The model under review builds one solid part; all positions refer to its coordinate system, in mm. A direction names the side the tool comes from. Coordinates: 2 decimals unless noted, no trailing zeros. Loops run counter-clockwise (first coordinate to the right, second up) from the corner with the lowest first, then second, coordinate; pieces in that order, holes last. Notation, with made-up numbers: (44, 3) - (49, 3) arc R22 cw to (49, 37) - close; hole circle Ø9 at (69, 69.5). An arc over 180 degrees is marked (long way). Use a Markdown table: item, result. Add a question column.
1) Clearance check with flat-ended pins moving along their axes: pin 1 (3 mm diameter, centred on x = -32.86, z = -52.86, fed in from -Y); pin 2 (2.5 mm diameter, centred on x = -2.8, z = -22.8, fed in from -Y); pin 3 (3 mm diameter, centred on x = -19.5, y = -46.5, fed in from +Z); pin 4 (24.5 mm diameter, centred on x = -0.5, z = -19.5, fed in from -Y). State where each tip first meets the part, or that it passes through.
2) Add section A-A, the plane x = 4.5. Give the boundary of the cut face in (y, z).
3) To check wall thickness, follow L1, parallel to X at y = -45.85, z = -27; L2, parallel to X at y = -44.6, z = -43.5; L3, parallel to Y at x = 3.5, z = -25.5. State the ranges of each line that lie inside material, in increasing order. Write a range as [from, to].
4) Add section B-B, the plane z = -20. Give the boundary of the cut face in (x, y).
5) Add section D-D, the plane z = -27. Give the boundary of the cut face in (x, y), and give its area (3 significant figures).
6) For faces 1 (the cylindrical face through (-5.189, -45.521, -25.505)), 2 (the cylindrical face through (8.1, -42.48, -21.85)), list the 3-axis set-ups (+Z, -Z, +X, -X, +Y, -Y) from which the entire face can be reached by the end or side of a thin tool; tool diameter is ignored.
7) Add section C-C, the plane y = -42.5. Give the number of separate pieces and of enclosed holes in the cut face, and give its area (3 significant figures).
8) The part is to be moulded in two halves that separate along X. For faces 3 (the flat face through (-7.152, -44.042, -42.708)), 4 (the cylindrical face through (8.479, -42.479, -12.934)), 5 (the cylindrical face through (10.105, -42.521, -9.553)), say which applies: pulls with the +X half, pulls with the -X half, needs draft (parallel to the pull), parting line crosses it, or undercut.
```python
from build123d import *

# Parameters (mm, degrees)
CYLINDER020_R             = 11.1
CYLINDER020_DEPTH         = 26
CYLINDER019_R             = 4
CYLINDER019_DEPTH         = 43
CYLINDER021_R             = 1
CYLINDER021_DEPTH         = 31
CYLINDER024_R             = 1
CYLINDER024_DEPTH         = 31
CYLINDER023_R             = 1
CYLINDER023_DEPTH         = 31
CYLINDER022_R             = 1
CYLINDER022_DEPTH         = 31
FUSION002_ROLL_ANGLE      = -90
FUSION003_PLACEMENT_ANGLE = 180
SKETCH_R                  = 5
SKETCH_R_2                = 1.75
PAD_DEPTH                 = 6
CUT_PITCH_ANGLE           = 90
CLONE017_PITCH_ANGLE      = -45


with BuildPart() as cylinder141:
    # Cylinder020 → Cylinder020 (new body)
    with BuildSketch(Plane(origin=(-3, 71, 73), x_dir=(0, 0, 1), z_dir=(0, -1, 0))):
        Circle(CYLINDER020_R)
    extrude(amount=CYLINDER020_DEPTH)


with BuildPart() as fusion001:
    # Cylinder019 → Cylinder019 (new body)
    with BuildSketch(Plane(origin=(-3, 66, 73), x_dir=(0, 0, 1), z_dir=(0, -1, 0))):
        Circle(CYLINDER019_R)
    extrude(amount=CYLINDER019_DEPTH)

    # Fusion001: union Cylinder141
    add(cylinder141.part)


with BuildPart() as cylinder096:
    # Cylinder021 → Cylinder021 (new body)
    with BuildSketch(Plane(origin=(-7.5, -11, 132), x_dir=(1, 0, 0), z_dir=(0, 0, 1))):
        Circle(CYLINDER021_R)
    extrude(amount=CYLINDER021_DEPTH)


with BuildPart() as cylinder146:
    # Cylinder024 → Cylinder024 (new body)
    with BuildSketch(Plane(origin=(0, -3.5, 132), x_dir=(1, 0, 0), z_dir=(0, 0, 1))):
        Circle(CYLINDER024_R)
    extrude(amount=CYLINDER024_DEPTH)


with BuildPart() as cylinder145:
    # Cylinder023 → Cylinder023 (new body)
    with BuildSketch(Plane(origin=(7.5, -11, 132), x_dir=(1, 0, 0), z_dir=(0, 0, 1))):
        Circle(CYLINDER023_R)
    extrude(amount=CYLINDER023_DEPTH)


with BuildPart() as fusion003:
    # Cylinder022 → Cylinder022 (new body)
    with BuildSketch(Plane(origin=(0, -18.5, 132), x_dir=(1, 0, 0), z_dir=(0, 0, 1))):
        Circle(CYLINDER022_R)
    extrude(amount=CYLINDER022_DEPTH)

    # Fusion002: union Cylinder096, Cylinder146, Cylinder145
    add(cylinder096.part)
    add(cylinder146.part)
    add(cylinder145.part)


with BuildPart() as fusion003_1:
    # Fusion002 roll: moved
    add(fusion003.part.rotate(Axis((0, 0, 0), (1, 0, 0)), FUSION002_ROLL_ANGLE))


with BuildPart() as fusion003_2:
    # Fusion002 placement: moved
    add(fusion003_1.part.moved(Location((-3, -97.5, 62))))

    # Fusion003: union Fusion001
    add(fusion001.part)


with BuildPart() as fusion003_3:
    # Fusion003 placement: moved
    add(fusion003_2.part.moved(Location((-0.5, 88, -87))).rotate(Axis((-0.5, 88, -87), (0, 0, 1)), FUSION003_PLACEMENT_ANGLE))


with BuildPart() as clone_of_cut001:
    # Sketch → Pad (new body)
    with BuildSketch(Plane(origin=(-11.5, 40, -16.5), x_dir=(0, 0, -1), z_dir=(0, 1, 0))):
        with BuildLine():
            Line((-2.5, -3), (47.5, -3))
            ThreePointArc((47.5, -25), (58.5, -14), (47.5, -3))
            Line((-2.5, -25), (47.5, -25))
            ThreePointArc((-2.5, -3), (-13.5, -14), (-2.5, -25))
        make_face()
        with Locations((14.166667, -14)):
            Circle(SKETCH_R, mode=Mode.SUBTRACT)
        with Locations((30.833333, -14)):
            Circle(SKETCH_R, mode=Mode.SUBTRACT)
        with Locations((47.5, -14)):
            Circle(SKETCH_R_2, mode=Mode.SUBTRACT)
    extrude(amount=PAD_DEPTH)

    # Cut: cut Fusion003
    add(fusion003_3.part, mode=Mode.SUBTRACT)


with BuildPart() as clone_of_cut001_1:
    # Cut pitch: moved
    add(clone_of_cut001.part.rotate(Axis((0, 0, 0), (0, 1, 0)), CUT_PITCH_ANGLE))


with BuildPart() as clone_of_cut001_2:
    # Cut placement: moved
    add(clone_of_cut001_1.part.moved(Location((16.5, -87, -15))))


with BuildPart() as clone_of_cut001_3:
    # Clone017 pitch: moved
    add(clone_of_cut001_2.part.rotate(Axis((0, 0, 0), (0, 1, 0)), CLONE017_PITCH_ANGLE))


with BuildPart() as clone_of_cut001_4:
    # Clone017 placement: moved
    add(clone_of_cut001_3.part.moved(Location((-11.642136, 0, -6.893398))))


solid = clone_of_cut001_4.part
```
From the geometry:
| question | item | result |
|---|---|---|
| 1 | pin 1 | passes through |
| 1 | pin 2 | stops at y = -44 |
| 1 | pin 3 | stops at z = -22.44 |
| 1 | pin 4 | stops at y = -47 |
| 2 | outline | (-47, -31.06) - (-41, -31.06) - (-41, -20.96) - (-44, -20.96) - (-44, -28.42) - (-47, -28.42) - close; (-44, -14.04) - (-41, -14.04) - (-41, -6.68) - (-44, -6.68) - close |
| 3 | L1 | x = [-22.56, -13.73], [-4.84, -3.24], [8.24, 8.56] |
| 3 | L2 | x = [-39.06, -25.44], [-16.7, -7.94] |
| 3 | L3 | y = [-44, -41] |
| 4 | outline | (-15.56, -47) - (-8.31, -47) - (-8.31, -44) - (-0.62, -44) - (-0.62, -41) - (-15.56, -41) - close; (5.62, -44) - (13.21, -44) - (13.21, -41) - (5.62, -41) - close |
| 5 | outline | (-22.56, -47) - (-13.73, -47) - (-13.73, -41) - (-22.56, -41) - close; (-4.84, -47) - (-3.24, -47) - (-3.24, -44) - (8.24, -44) - (8.24, -47) - (8.56, -47) - (8.56, -41) - (-4.84, -41) - close |
| 5 | area | 98.9 mm^2 |
| 6 | face 1 | -Y |
| 6 | face 2 | +Y, -Y |
| 7 | separate pieces | 1 |
| 7 | enclosed holes | 8 |
| 7 | area | 1,250 mm^2 |
| 8 | face 3 | pulls with the +X half |
| 8 | face 4 | undercut |
| 8 | face 5 | parting line crosses it |
